from build123d import *

# Parameters (mm, degrees)
F1_W     = 83.3939239383
F1_H     = 70.5358162522
F1_R     = 18.1915256805
F2_DEPTH = 107.3792502284
F3_W     = 68.390481174
F3_H     = 34.5757827163
F4_DEPTH = 190.568074584
F5_DEPTH = 25.4


with BuildPart() as f2:
    # F1 (on face) → F2 (new body)
    with BuildSketch(Plane.XZ):
        with Locations((-1.7756335437, 1.8368847668)):
            Rectangle(F1_W, F1_H)
        with Locations((13.2254809141, 12.4907270074)):
            Circle(F1_R, mode=Mode.SUBTRACT)
    extrude(amount=F2_DEPTH)

    # F3 (on face) → F4 (join)
    with BuildSketch(Plane(origin=(-43.4725955129, 0, 0), x_dir=(0, -1, 0), z_dir=(-1, 0, 0))):
        with Locations((55.904109031, 1.3973750174)):
            Rectangle(F3_W, F3_H)
    extrude(amount=-F4_DEPTH)

    # F5 (add): a face of the model
    f5_faces = [f2.faces().sort_by_distance(p)[0] for p in [
        (93.5084037483, -55.904109031, 18.6852663755),
    ]]
    extrude(f5_faces, amount=F5_DEPTH)


solid = f2.part
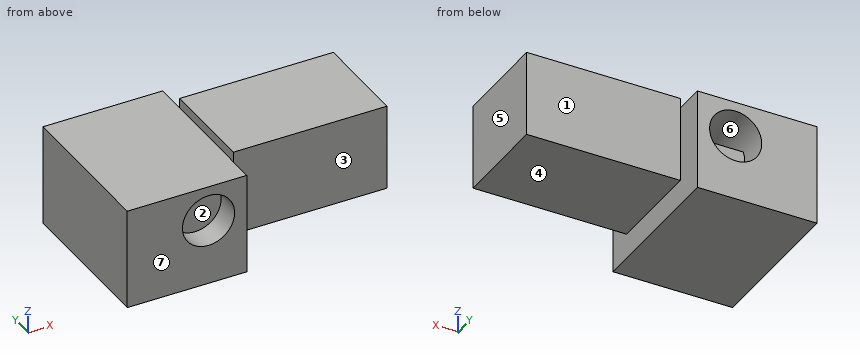
Design review of the part built by this model. Coordinates are the model's own, in mm. Face numbers are marked on the shaded views. A direction names the side the tool comes from. Coordinates: 2 decimals unless noted, no trailing zeros. Order: outer loops, then holes, each group sorted by start corner. A loop starts at its lowest first (then second) coordinate and runs counter-clockwise, first axis right, second up.
Item 1: The part is to be moulded in two halves that separate along X. For the marked faces 5, 6 and 7, say which applies: pulls with the +X half, pulls with the -X half, needs draft (parallel to the pull), parting line crosses it, or undercut.
Item 2: Take a section at C-C, the plane z = 5. Write out the cut boundary in (x, y).
Item 3: Take a section at B-B, the plane x = 24. Write out the cut boundary in (y, z), then the cut area to 3 significant figures.
Item 4: Take a section at D-D, the plane x = 111. Write out the cut boundary in (y, z).
Item 5: For the marked faces 1, 2, 3 and 4, list the 3-axis set-ups (+Z, -Z, +X, -X, +Y, -Y) from which the entire face can be reached by the end or side of a thin tool; tool diameter is ignored.
Item 6: For pin 1 Ø4 at (x, z) = (122, 11.5) entering from -Y; pin 2 Ø3 at (x, z) = (125, 27) entering from +Y; pin 3 Ø3 at (x, y) = (80.5, -68) entering from -Z, all flat-tipped, find the tip position at first contact; note any pin that passes through.
Item 7: For line 1 (Z direction, x = 12.5, y = -19); line 2 (Y direction, x = 132.5, z = 18); line 3 (Z direction, x = 105.5, y = -26.5), list the stretches that pass through material, from the lowest coordinate up.
Item 8: Take a section at A-A, the plane y = -86. Write out the cut boundary in (x, z), then the cut area to 3 significant figures.
The answers:
1. face 5: pulls with the +X half
1. face 6: undercut
1. face 7: needs draft
2. outline: (-43.47, -107.38) - (-3.35, -107.38) - (-3.35, -90.1) - (29.8, -90.1) - (29.8, -107.38) - (39.92, -107.38) - (39.92, -90.1) - (147.1, -90.1) - (147.1, -21.71) - (39.92, -21.71) - (39.92, 0) - (29.8, 0) - (29.8, -21.71) - (-3.35, -21.71) - (-3.35, 0) - (-43.47, 0) - close
3. outline: (-107.38, -33.43) - (0, -33.43) - (0, -2.17) - (-21.71, -2.17) - (-21.71, 18.69) - (-90.1, 18.69) - (-90.1, -2.17) - (-107.38, -2.17) - close; (-107.38, 27.15) - (0, 27.15) - (0, 37.1) - (-107.38, 37.1) - close
3. area: 5,850 mm2
4. outline: (-90.1, -15.89) - (-21.71, -15.89) - (-21.71, 44.09) - (-90.1, 44.09) - close
5. face 1: +Z, -Z, +X, +Y
5. face 2: -Y
5. face 3: +Z, -Z, +X, -Y
5. face 4: -Z, +X, +Y, -Y
6. pin 1: stops at y = -90.1
6. pin 2: stops at y = -21.71
6. pin 3: stops at z = -15.89
7. line 1: z = -33.43 to -5.69, 30.67 to 37.1
7. line 2: y = -90.1 to -21.71
7. line 3: z = -15.89 to 44.09
8. outline: (-43.47, -33.43) - (39.92, -33.43) - (39.92, -15.89) - (147.1, -15.89) - (147.1, 44.09) - (39.92, 44.09) - (39.92, 37.1) - (-43.47, 37.1) - close; hole (-3.88, 18.69) - (30.33, 18.69) arc R18.19 ccw to start
8. area: 12,000 mm2
